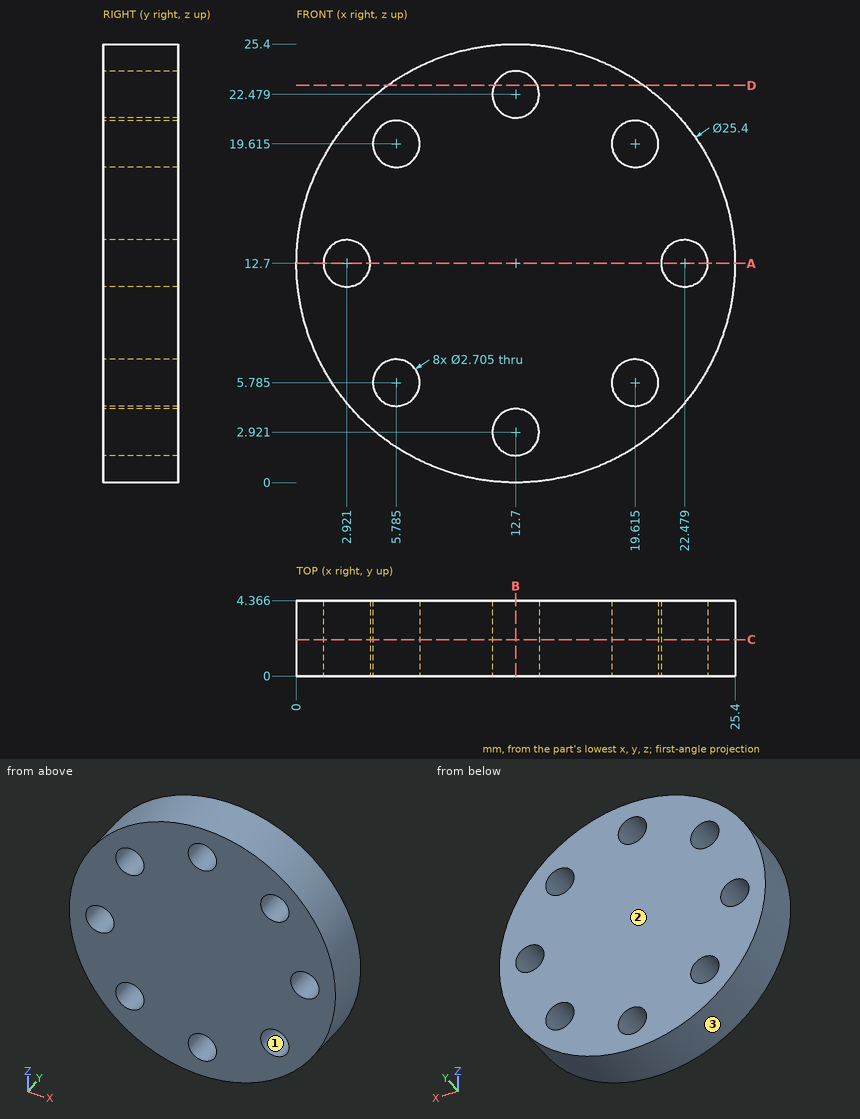
Could you check a few things on this drawing? It's one solid part, dimensions in mm from its lowest x, y, z. Round coordinates to 2 decimals unless told otherwise and drop trailing zeros. Loops run counter-clockwise (first coordinate to the right, second up) from the corner with the lowest first, then second, coordinate; pieces in that order, holes last.
Q1. I want a section at D-D (z = 23). Write out the boundary of the cut face in (x, y) (1 decimal).
Q2. Thinking about a two-plate mould opening in Z: for the marked faces 1, 2 and 3, which applies, pulls with the +Z half, pulls with the -Z half, needs draft (parallel to the pull), parting line crosses it, or undercut?
Q3. I want a section at B-B (x = 12.7). Write out the boundary of the cut face in (y, z) (1 decimal).
Q4. For P1, Ø2, axis at y = 0.5, z = 15, coming from the +X side; P2, Ø2.5, axis at x = 12.7, z = 22.479, coming from the -Y side; P3, Ø1, axis at x = 22, y = 3, coming from the +Z side; P4, Ø1, axis at y = 2, z = 15.5, coming from the -X side, each with a flat end and sliding along its axis, tell me the tip position at first contact or that it passes through.
Q5. Please list where these lines run through material, in increasing order: L1, parallel to X at y = 3, z = 12.7; L2, parallel to Z at x = 13, y = 2.8; L3, parallel to Z at x = 11.5, y = 2.25 (1 decimal).
Q6. I want a section at C-C (y = 2.1). Give the number of separate pieces and of enclosed holes in the cut face, and give its area (3 significant figures).
Q7. I want a section at A-A (z = 12.7). Write out the boundary of the cut face in (x, y) (1 decimal).
Answer below:
1. outline: (5.3, 0) - (11.5, 0) - (11.5, 4.4) - (5.3, 4.4) - close; (13.9, 0) - (20.1, 0) - (20.1, 4.4) - (13.9, 4.4) - close
2. face 1: undercut
2. face 2: needs draft
2. face 3: parting line crosses it
3. outline: (0, 0) - (4.4, 0) - (4.4, 1.6) - (0, 1.6) - close; (0, 4.3) - (4.4, 4.3) - (4.4, 21.1) - (0, 21.1) - close; (0, 23.8) - (4.4, 23.8) - (4.4, 25.4) - (0, 25.4) - close
4. P1: stops at x = 25.33
4. P2: passes through
4. P3: stops at z = 21.86
4. P4: stops at x = 0.21
5. L1: x = 0 to 1.57, 4.27 to 21.13, 23.83 to 25.4
5. L2: z = 0 to 1.6, 4.24 to 21.16, 23.8 to 25.4
5. L3: z = 0.1 to 2.3, 3.5 to 21.9, 23.1 to 25.3
6. separate pieces: 1
6. enclosed holes: 8
6. area: 461 mm2
7. outline: (0, 0) - (1.6, 0) - (1.6, 4.4) - (0, 4.4) - close; (4.3, 0) - (21.1, 0) - (21.1, 4.4) - (4.3, 4.4) - close; (23.8, 0) - (25.4, 0) - (25.4, 4.4) - (23.8, 4.4) - close
